Part model, mm, in its own coordinate system. Face numbers are marked on the shaded views. A direction names the side the tool comes from. Coordinates: 2 decimals unless noted, no trailing zeros. Order: outer loops, then holes, each group sorted by start corner. A loop starts at its lowest first (then second) coordinate and runs counter-clockwise, first axis right, second up.
from build123d import *

# Parameters (mm, degrees)
SKETCH1_R           = 32.5
SKETCH1_R_2         = 2.65
SKETCH1_R_3         = 11.1
BOSS_EXTRUDE1_DEPTH = 3
SKETCH2_R           = 4.65
SKETCH2_R_2         = 2.65
BOSS_EXTRUDE2_DEPTH = 2
SKETCH3_R           = 32.5
SKETCH3_R_2         = 11.1
SKETCH3_R_3         = 4.25
BOSS_EXTRUDE3_DEPTH = 7
SKETCH4_R           = 11.1
SKETCH4_R_2         = 1.5
BOSS_EXTRUDE4_DEPTH = 2.5
SKETCH5_R           = 1.5
CUT_EXTRUDE1_DEPTH  = 13
SKETCH6_R           = 6
CUT_EXTRUDE2_DEPTH  = 1


with BuildPart() as part:
    # Sketch1 → Boss-Extrude1 (new body)
    with BuildSketch(Plane(origin=(0, 0, 0), x_dir=(1, 0, 0), z_dir=(0, 1, 0))):
        Circle(SKETCH1_R)
        with Locations((0, 27.5)):
            Circle(SKETCH1_R_2, mode=Mode.SUBTRACT)
        with Locations((27.5, 0)):
            Circle(SKETCH1_R_2, mode=Mode.SUBTRACT)
        with Locations((0, -27.5)):
            Circle(SKETCH1_R_2, mode=Mode.SUBTRACT)
        with Locations((-27.5, 0)):
            Circle(SKETCH1_R_2, mode=Mode.SUBTRACT)
        Circle(SKETCH1_R_3, mode=Mode.SUBTRACT)
    extrude(amount=BOSS_EXTRUDE1_DEPTH)

    # Sketch2 → Boss-Extrude2 (add)
    with BuildSketch(Plane(origin=(0, 3, 0), x_dir=(1, 0, 0), z_dir=(0, 1, 0))):
        with Locations((0, -27.5)):
            Circle(SKETCH2_R)
        with Locations((0, -27.5)):
            Circle(SKETCH2_R_2, mode=Mode.SUBTRACT)
        with Locations((27.5, 0)):
            Circle(SKETCH2_R)
        with Locations((27.5, 0)):
            Circle(SKETCH2_R_2, mode=Mode.SUBTRACT)
        with Locations((0, 27.5)):
            Circle(SKETCH2_R)
        with Locations((0, 27.5)):
            Circle(SKETCH2_R_2, mode=Mode.SUBTRACT)
        with Locations((-27.5, 0)):
            Circle(SKETCH2_R)
        with Locations((-27.5, 0)):
            Circle(SKETCH2_R_2, mode=Mode.SUBTRACT)
    extrude(amount=BOSS_EXTRUDE2_DEPTH)

    # Sketch3 → Boss-Extrude3 (add)
    with BuildSketch(Plane(origin=(0, 0, 0), x_dir=(-1, 0, 0), z_dir=(0, -1, 0))):
        Circle(SKETCH3_R)
        Circle(SKETCH3_R_2, mode=Mode.SUBTRACT)
        with Locations((0, 27.5)):
            Circle(SKETCH3_R_3, mode=Mode.SUBTRACT)
        with Locations((27.5, 0)):
            Circle(SKETCH3_R_3, mode=Mode.SUBTRACT)
        with Locations((0, -27.5)):
            Circle(SKETCH3_R_3, mode=Mode.SUBTRACT)
        with Locations((-27.5, 0)):
            Circle(SKETCH3_R_3, mode=Mode.SUBTRACT)
    extrude(amount=BOSS_EXTRUDE3_DEPTH)

    # Sketch4 → Boss-Extrude4 (add)
    with BuildSketch(Plane(origin=(0, -7, 0), x_dir=(-1, 0, 0), z_dir=(0, -1, 0))):
        Circle(SKETCH4_R)
        with Locations((0, 8)):
            Circle(SKETCH4_R_2, mode=Mode.SUBTRACT)
        with Locations((8, 0)):
            Circle(SKETCH4_R_2, mode=Mode.SUBTRACT)
        with Locations((0, -8)):
            Circle(SKETCH4_R_2, mode=Mode.SUBTRACT)
        with Locations((-8, 0)):
            Circle(SKETCH4_R_2, mode=Mode.SUBTRACT)
    extrude(amount=-BOSS_EXTRUDE4_DEPTH)

    # Sketch5 → Cut-Extrude1 (cut, through all)
    with BuildSketch(Plane.XZ.offset(7)):
        with Locations((0, 16)):
            Circle(SKETCH5_R)
        with Locations((8, 13.856406461)):
            Circle(SKETCH5_R)
        with Locations((13.856406461, 8)):
            Circle(SKETCH5_R)
        with Locations((16, 0)):
            Circle(SKETCH5_R)
        with Locations((13.856406461, -8)):
            Circle(SKETCH5_R)
        with Locations((8, -13.856406461)):
            Circle(SKETCH5_R)
        with Locations((0, -16)):
            Circle(SKETCH5_R)
        with Locations((-8, -13.856406461)):
            Circle(SKETCH5_R)
        with Locations((-13.856406461, -8)):
            Circle(SKETCH5_R)
        with Locations((-16, 0)):
            Circle(SKETCH5_R)
        with Locations((-13.856406461, 8)):
            Circle(SKETCH5_R)
        with Locations((-8, 13.856406461)):
            Circle(SKETCH5_R)
    extrude(amount=-CUT_EXTRUDE1_DEPTH, mode=Mode.SUBTRACT)

    # Sketch6 → Cut-Extrude2 (cut)
    with BuildSketch(Plane(origin=(0, -4.5, 0), x_dir=(1, 0, 0), z_dir=(0, 1, 0))):
        Circle(SKETCH6_R)
    extrude(amount=-CUT_EXTRUDE2_DEPTH, mode=Mode.SUBTRACT)


solid = part.part
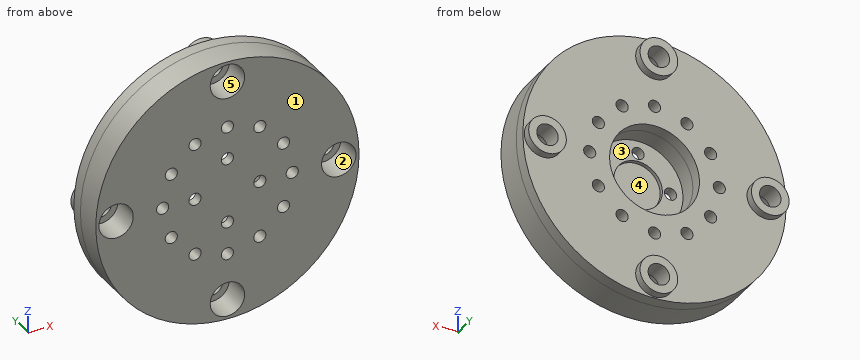
Q1. Mould opens along X. For the marked faces 1, 2 and 3 say: pulls with the +X half, pulls with the -X half, needs draft (parallel to the pull), parting line crosses it, or undercut.
Results list:
face 1: needs draft
face 2: undercut
face 3: undercut
Q2. Pin check, flat tips, straight feed: pin 1 Ø4 at (x, z) = (-0.5, -27) entering from -Y; pin 2 Ø4 at (x, z) = (4.5, 5.5) entering from +Y; pin 3 Ø9.5 at (x, z) = (0, 0) entering from +Y. Stop position of each tip, or through.
Results list:
pin 1: stops at y = 0
pin 2: stops at y = -4.5
pin 3: stops at y = -5.5
Q3. Cut at D-D on z = -8. Write the cut outline in (x, y).
Results list:
outline: (-31.5, -7) - (-15.36, -7) - (-15.36, 3) - (-31.5, 3) - close; (-12.36, -7) - (-1.5, -7) - (-1.5, -4.5) - (-7.69, -4.5) - (-7.69, 3) - (-12.36, 3) - close; (1.5, -7) - (12.36, -7) - (12.36, 3) - (7.69, 3) - (7.69, -4.5) - (1.5, -4.5) - close; (15.36, -7) - (31.5, -7) - (31.5, 3) - (15.36, 3) - close
Q4. Cut at A-A on z = -27.5. Write the cut outline in (x, y), and give its area (3 significant figures).
Results list:
outline: (-17.32, -7) - (-4.25, -7) - (-4.25, 0) - (-2.65, 0) - (-2.65, 5) - (-4.65, 5) - (-4.65, 3) - (-17.32, 3) - close; (2.65, 0) - (4.25, 0) - (4.25, -7) - (17.32, -7) - (17.32, 3) - (4.65, 3) - (4.65, 5) - (2.65, 5) - close
area: 279 mm2
Q5. Cut at C-C on x = 13.5. Write the cut outline in (y, z), and give its area (3 significant figures).
Results list:
outline: (-7, -29.56) - (3, -29.56) - (3, -9.46) - (-7, -9.46) - close; (-7, -6.54) - (3, -6.54) - (3, 6.54) - (-7, 6.54) - close; (-7, 9.46) - (3, 9.46) - (3, 29.56) - (-7, 29.56) - close
area: 533 mm2
Q6. Which spindle directions (+Z, -Z, +X, -X, +Y, -Y) get a long thin tool onto all of the face, cutting with end or side? Do the marked faces 4 and 5. Say none if no direction does.
Results list:
face 4: +Y
face 5: -Y
Q7. Wall check: line 1 along X through (y, z) = (-4, -13); line 2 along X through (y, z) = (0.25, -0.5); line 3 along Z through (x, y) = (2.5, -6). Give the ranges that are in metal, low to high.
Results list:
line 1: x = -29.79 to -9.23, -6.77 to 6.77, 9.23 to 29.79
line 2: x = -32.5 to -30.1, -24.9 to -17.41, -14.59 to -11.09, 11.09 to 14.59, 17.41 to 24.9, 30.1 to 32.5
line 3: z = -32.4 to -30.94, -24.06 to 24.06, 30.94 to 32.4
Q8. Cut at B-B on x = -16.5. Write the cut outline in (y, z).
Results list:
outline: (-7, -28) - (3, -28) - (3, -1.41) - (-7, -1.41) - close; (-7, 1.41) - (3, 1.41) - (3, 28) - (-7, 28) - close
